Input: part model. Units: mm. Frame: model coordinates. Face numbers are marked on the shaded views. A direction names the side the tool comes from. Give positions to 0.01 mm unless a question says otherwise; leave off trailing zeros. Loops run counter-clockwise (first coordinate to the right, second up) from the corner with the lowest first, then second, coordinate; pieces in that order, holes last. Notation, with made-up numbers: (11, 47.25) - (37, 47.25) arc R30 cw to (37, 77.25) - close; hole circle Ø5 at (72.25, -28.5). An arc over 180 degrees is marked (long way). Answer as a JSON object with one key per item and string values. Group by question number.
(1) Material intervals for L1, parallel to Y at x = 0, z = 2; L2, parallel to Z at x = 41.5, y = -40; L3, parallel to Z at x = 16, y = -35, sorted ascending.
(2) Pin query (flat end, axial travel): P1, Ø12, axis at x = -9, z = -16.5, coming from the -Y side; P2, Ø16.5, axis at x = 47.62, y = 42, coming from the -Z side; P3, Ø12, axis at y = 49.5, z = -19.5, coming from the -X side. Return the tip coordinate at first contact, or that it passes through.
(3) Mould query, pull axis Y, two halves, no side actions, for the marked faces 1, 2, 3 and 4. Classes: +Y half, -Y half, draft (parallel to the pull), parting line (faces both ways), or undercut.
(4) Section query A-A (x = 0). Return loops of the section in (y, z).
(5) Section query D-D (x = 63.5). Return loops of the section in (y, z).
(6) Section query C-C (z = -17). Return loops of the section in (x, y), plus the area to 3 significant figures.
(7) Access query for the marked faces 5 and 6. Directions: +Z, -Z, +X, -X, +Y, -Y. A direction counts if a zero-diameter tool reaches every point of the face in a straight line with its end or side. Return the directions, or none.
```python
from build123d import *

# Parameters (mm, degrees)
F0_R     = 50.8
F0_R_2   = 38.1
F1_DEPTH = 31.75
F0_R_3   = 76.2
F0_R_4   = 6.35
F2_DEPTH = 6.35


with BuildPart() as f1:
    # F0 (on Top) → F1 (new body)
    with BuildSketch(Plane.XY):
        Circle(F0_R)
        Circle(F0_R_2, mode=Mode.SUBTRACT)
    extrude(amount=-F1_DEPTH)

    # F0 (on Top) → F2 (join, symmetric)
    with BuildSketch(Plane.XY):
        Circle(F0_R_3)
        with Locations((-47.502615, -42.139667)):
            Circle(F0_R_4, mode=Mode.SUBTRACT)
        with Locations((0, -63.5)):
            Circle(F0_R_4, mode=Mode.SUBTRACT)
        with Locations((47.622745, -42.003859)):
            Circle(F0_R_4, mode=Mode.SUBTRACT)
        with Locations((-63.5, 0)):
            Circle(F0_R_4, mode=Mode.SUBTRACT)
        with Locations((-45.076814, 44.725058)):
            Circle(F0_R_4, mode=Mode.SUBTRACT)
        Circle(F0_R, mode=Mode.SUBTRACT)
        with Locations((63.5, 0)):
            Circle(F0_R_4, mode=Mode.SUBTRACT)
        with Locations((0, 63.5)):
            Circle(F0_R_4, mode=Mode.SUBTRACT)
        with Locations((47.622745, 42.003859)):
            Circle(F0_R_4, mode=Mode.SUBTRACT)
    extrude(amount=F2_DEPTH, both=True)


solid = f1.part
```
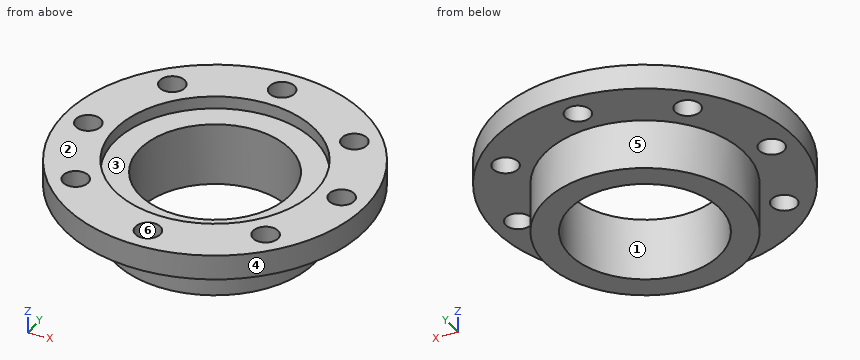
Recorded:
{
 "1": {"L1": "y = -76.2 to -69.85, -57.15 to -50.8, 50.8 to 57.15, 69.85 to 76.2", "L2": "z = -6.35 to 6.35", "L3": "z = -31.75 to 0"},
 "2": {"P1": "stops at y = -50.71", "P2": "stops at z = -6.35", "P3": "stops at x = -26.24"},
 "3": {"face 1": "undercut", "face 2": "draft", "face 3": "undercut", "face 4": "parting line"},
 "4": {"outline": "(-76.2, -6.35) - (-69.85, -6.35) - (-69.85, 6.35) - (-76.2, 6.35) - close; (-57.15, -6.35) - (-50.8, -6.35) - (-50.8, -31.75) - (-38.1, -31.75) - (-38.1, 0) - (-50.8, 0) - (-50.8, 6.35) - (-57.15, 6.35) - close; (38.1, -31.75) - (50.8, -31.75) - (50.8, -6.35) - (57.15, -6.35) - (57.15, 6.35) - (50.8, 6.35) - (50.8, 0) - (38.1, 0) - close; (69.85, -6.35) - (76.2, -6.35) - (76.2, 6.35) - (69.85, 6.35) - close"},
 "5": {"outline": "(-42.12, -6.35) - (-6.35, -6.35) - (-6.35, 6.35) - (-42.12, 6.35) - close; (6.35, -6.35) - (42.12, -6.35) - (42.12, 6.35) - (6.35, 6.35) - close"},
 "6": {"outline": "circle Ø101.6 at (0, 0); hole circle Ø76.2 at (0, 0)", "area": "3,550 mm^2"},
 "7": {"face 5": "-Z", "face 6": "+Z, -Z"}
}
